Geometry check sheet. Reference: drawing and pictorial views, mm from the part's lowest x, y, z. A direction names the side the tool comes from. Round coordinates to 2 decimals unless told otherwise and drop trailing zeros. Write each loop counter-clockwise with the first axis right and the second up, starting at its lowest first coordinate (ties: lowest second). Pieces come first, ordered by that corner, then holes. Notation, with made-up numbers: M 39,-6.75 L 82,-6.75 A13 cw 82,12.25 Z; hole C 66,63.25 d10. An arc over 180 degrees is marked long. Answer in a Markdown table with one row per item.
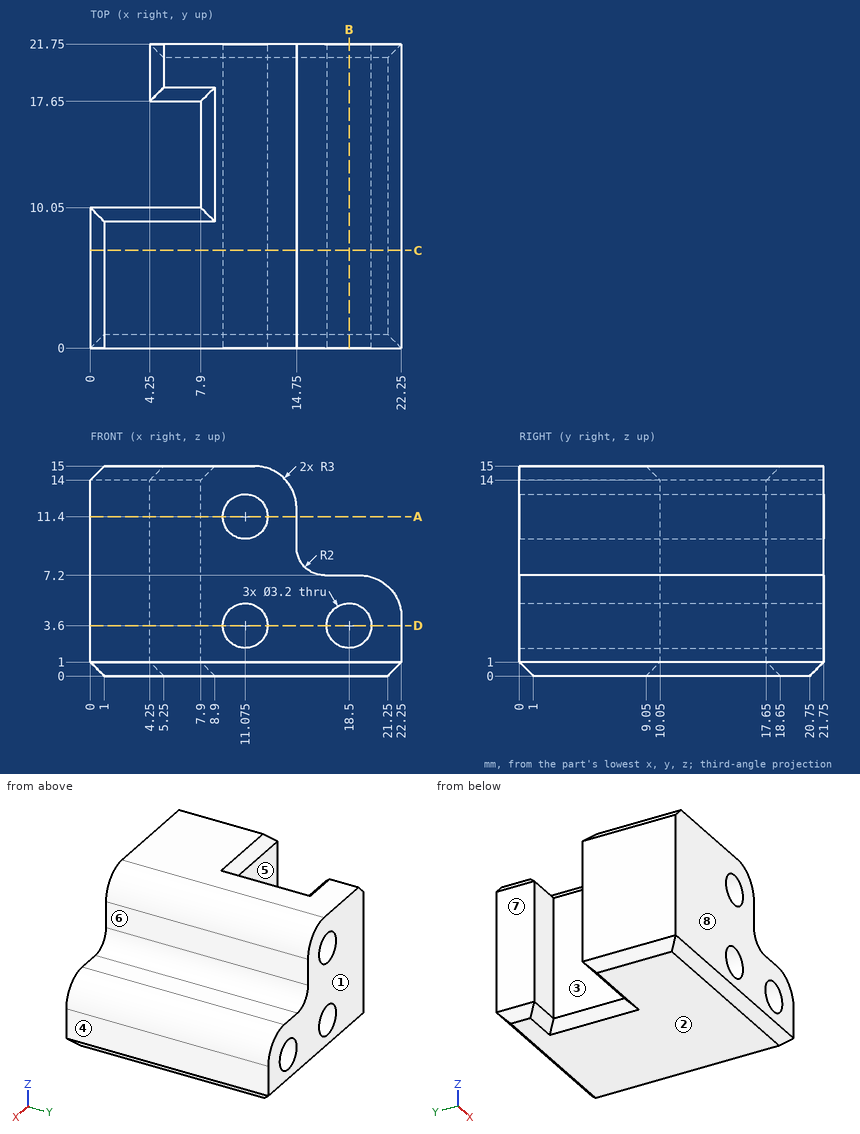
1. Go/stop test with flat-tipped pins: pin 1 (3 mm diameter, centred on x = 2.5, y = 13.5, fed in from -Z); pin 2 (6 mm diameter, centred on x = 17.5, y = 19, fed in from +Z); pin 3 (0.8 mm diameter, centred on y = 13, z = 10, fed in from +X); pin 4 (1.2 mm diameter, centred on y = 20, z = 5.5, fed in from -X). Record where each tip stops, or that it passes through.
Found:
| item | result |
|---|---|
| pin 1 | passes through |
| pin 2 | stops at z = 13.2 |
| pin 3 | stops at x = 14.75 |
| pin 4 | stops at x = 4.25 |
2. Draft check along Y on the marked faces 1, 2 and 3. Enter one of: +Y half, -Y half, draft (parallel to the pull), parting line (faces both ways), or undercut.
Found:
| item | result |
|---|---|
| face 1 | +Y half |
| face 2 | draft |
| face 3 | undercut |
3. Access from +Z, -Z, +X, -X, +Y, -Y to the whole of each face (thin tool, end or side, straight path). Record for the marked faces 4, 5, 6, 7 and 8.
Found:
| item | result |
|---|---|
| face 4 | +Z, -Z, +X, +Y, -Y |
| face 5 | +Z, -Z, -X |
| face 6 | +Z, +X, +Y, -Y |
| face 7 | +Z, -Z, -X, +Y |
| face 8 | +Z, -Z, +X, -X, -Y |
4. Section check A-A, the plane z = 11.4. Record the cut outline in (x, y) (3 decimals), and give its area (3 significant figures).
Found:
| item | result |
|---|---|
| outline | M 0,0 L 9.475,0 L 9.475,21.75 L 4.25,21.75 L 4.25,17.65 L 7.9,17.65 L 7.9,10.05 L 0,10.05 Z; M 12.675,0 L 14.75,0 L 14.75,21.75 L 12.675,21.75 Z |
| area | 174 mm2 |
5. Section check B-B, the plane x = 18.5. Record the cut outline in (y, z).
Found:
| item | result |
|---|---|
| outline | M 0,1 L 1,0 L 20.75,0 L 21.75,1 L 21.75,2 L 0,2 Z; M 0,5.2 L 21.75,5.2 L 21.75,7.2 L 0,7.2 Z |
6. Section check D-D, the plane z = 3.6. Record the cut outline in (x, y) (3 decimals), and give its area (3 significant figures).
Found:
| item | result |
|---|---|
| outline | M 0,0 L 9.475,0 L 9.475,21.75 L 4.25,21.75 L 4.25,17.65 L 7.9,17.65 L 7.9,10.05 L 0,10.05 Z; M 12.675,0 L 16.9,0 L 16.9,21.75 L 12.675,21.75 Z; M 20.1,0 L 22.25,0 L 22.25,21.75 L 20.1,21.75 Z |
| area | 267 mm2 |
7. Section check C-C, the plane y = 7. Record the cut outline in (x, z) (3 decimals).
Found:
| item | result |
|---|---|
| outline | M 0,1 L 1,0 L 21.25,0 L 22.25,1 L 22.25,4.2 A3 ccw 19.25,7.2 L 16.75,7.2 A2 cw 14.75,9.2 L 14.75,12 A3 ccw 11.75,15 L 1,15 L 0,14 Z; hole C 11.075,3.6 d3.2; hole C 11.075,11.4 d3.2; hole C 18.5,3.6 d3.2 |
8. Scan lines: L1, parallel to X at y = 9, z = 5; L2, parallel to X at y = 6, z = 4.75; L3, parallel to Y at x = 1.5, z = 10.75. Record each from-to range of solid material in increasing order.
Found:
| item | result |
|---|---|
| L1 | x = 0 to 10.3, 11.85 to 17.73, 19.27 to 22.14 |
| L2 | x = 0 to 9.96, 12.19 to 17.39, 19.61 to 22.2 |
| L3 | y = 0 to 10.05 |
